Verification items for the finished model (mm, model axes). Round coordinates to 2 decimals unless told otherwise and drop trailing zeros. Write each loop counter-clockwise with the first axis right and the second up, starting at its lowest first coordinate (ties: lowest second). Pieces come first, ordered by that corner, then holes. Notation, with made-up numbers: (23.5, -38) -> (55.5, -38) arc R26 ccw to (55.5, -14) -> close; hole circle Ø8 at (-31, -3). An arc over 180 degrees is marked (long way). Answer as a JSON object with one key per item and string values. Group by question number.
(1) Sectioned sample at D-D on z = -14.5. Record the cut outline in (x, y).
(2) Sectioned sample at A-A on z = -5.25. Record the cut outline in (x, y).
(3) Sectioned sample at B-B on x = 3.5. Record the cut outline in (y, z).
(4) Sectioned sample at C-C on y = -2.3. Record the cut outline in (x, z), and give its area (3 significant figures).
(5) Scan lines: L1, parallel to Z at x = -1, y = -0.5; L2, parallel to Z at x = 0.5, y = -2; L3, parallel to X at y = -1.55, z = -6.25. Record each from-to range of solid material in increasing order. Write a range as from..to.
(6) Gauge pin test, flat end, axial feed: pin 1 Ø1 at (x, y) = (-2, -1) entering from -Z. Record the tip position at first contact, or that the pin passes through.
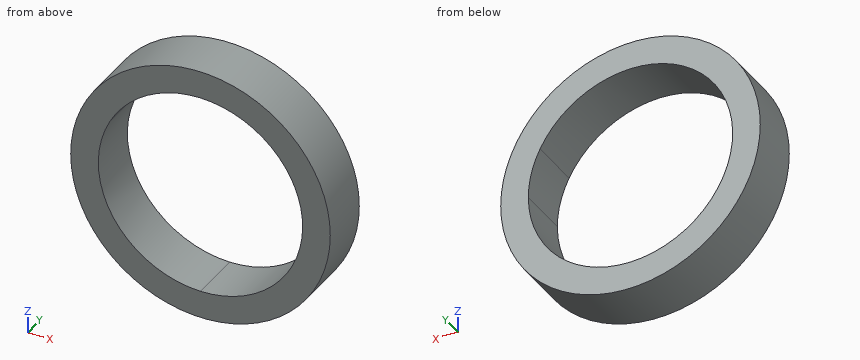
```python
from build123d import *

# Parameters (mm, degrees)
F0_R     = 6.35
F1_DEPTH = 2.54


# Not quite as in the source:
# - a feature names something its author has since deleted; it is built from what else it names


with BuildPart() as f1:
    # F0 (on Front) → F1 (new body)
    with BuildSketch(Plane.XZ):
        with Locations((0, -9.0619377949)):
            Circle(F0_R)
        with BuildLine():
            ThreePointArc((4.4250278693, -6.7369416578), (4.8531244574, -7.864581673), (4.9986476853, -9.0619377949))
            ThreePointArc((4.9986476853, -9.0619377949), (3.534577675, -12.59651547), (0, -14.0605854803))
            ThreePointArc((0, -14.0605854803), (-4.2732397818, -11.6553718984), (-4.434145585, -6.7543781288))
            ThreePointArc((-4.434145585, -6.7543781288), (-0.0098382323, -4.0632997914), (4.4250278693, -6.7369416578))
        make_face(mode=Mode.SUBTRACT)
    extrude(amount=F1_DEPTH)


solid = f1.part
```
Computed values:
{
 "1": {"outline": "(-3.28, -2.54) -> (3.28, -2.54) -> (3.28, 0) -> (-3.28, 0) -> close"},
 "2": {"outline": "(-5.08, -2.54) -> (-3.23, -2.54) -> (-3.23, 0) -> (-5.08, 0) -> close; (3.23, -2.54) -> (5.08, -2.54) -> (5.08, 0) -> (3.23, 0) -> close"},
 "3": {"outline": "(-2.54, -14.36) -> (0, -14.36) -> (0, -12.63) -> (-2.54, -12.63) -> close; (-2.54, -5.49) -> (0, -5.49) -> (0, -3.76) -> (-2.54, -3.76) -> close"},
 "4": {"outline": "circle Ø12.7 at (0, -9.06); hole circle Ø10 at (0, -9.06)", "area": "48.2 mm2"},
 "5": {"L1": "-15.33..-13.96, -4.16..-2.79", "L2": "-15.39..-14.04, -4.09..-2.73", "L3": "-5.69..-4.13, 4.13..5.69"},
 "6": {"pin 1": "z = -15.23"}
}
